from build123d import *

# Parameters (mm, degrees)
SKETCH1_R           = 5
BOSS_EXTRUDE1_DEPTH = 17
SKETCH2_R           = 5
SKETCH2_R_2         = 4
CUT_EXTRUDE1_DEPTH  = 12
CUT_EXTRUDE2_START  = -4
SKETCH3_R           = 4
SKETCH3_R_2         = 3.5
CUT_EXTRUDE2_DEPTH  = 1
SKETCH4_R           = 4
BOSS_EXTRUDE2_DEPTH = 6


with BuildPart() as part:
    # Sketch1 → Boss-Extrude1 (new, symmetric)
    with BuildSketch(Plane(origin=(0, 0, 0), x_dir=(1, 0, 0), z_dir=(0, 1, 0))):
        with Locations(Location((0, 0, 0), (0, 0, 270))):
            Circle(SKETCH1_R)
    extrude(amount=BOSS_EXTRUDE1_DEPTH, both=True)

    # Sketch2 → Cut-Extrude1 (cut)
    with BuildSketch(Plane(origin=(0, 17, 0), x_dir=(1, 0, 0), z_dir=(0, 1, 0))):
        with Locations(Location((0, 0, 0), (0, 0, 270))):
            Circle(SKETCH2_R)
        with Locations(Location((0, 0, 0), (0, 0, 270))):
            Circle(SKETCH2_R_2, mode=Mode.SUBTRACT)
    cut_extrude1 = extrude(amount=-CUT_EXTRUDE1_DEPTH, mode=Mode.SUBTRACT)

    # Mirror1: Cut-Extrude1 across plane
    add(cut_extrude1.mirror(Plane.ZX), mode=Mode.SUBTRACT)

    # Sketch3 → Cut-Extrude2 (cut)
    with BuildSketch(Plane(origin=(0, 17, 0), x_dir=(1, 0, 0), z_dir=(0, 1, 0)).offset(CUT_EXTRUDE2_START)):
        with Locations(Location((0, 0, 0), (0, 0, 270))):
            Circle(SKETCH3_R)
        with Locations(Location((0, 0, 0), (0, 0, 270))):
            Circle(SKETCH3_R_2, mode=Mode.SUBTRACT)
    cut_extrude2 = extrude(amount=-CUT_EXTRUDE2_DEPTH, mode=Mode.SUBTRACT)

    # Mirror2: Cut-Extrude2 across plane
    add(cut_extrude2.mirror(Plane.ZX), mode=Mode.SUBTRACT)

    # Sketch4 → Boss-Extrude2 (add)
    with BuildSketch(Plane(origin=(0, 17, 0), x_dir=(1, 0, 0), z_dir=(0, 1, 0))):
        with Locations(Location((0, 0, 0), (0, 0, 270))):
            Circle(SKETCH4_R)
    extrude(amount=BOSS_EXTRUDE2_DEPTH)


solid = part.part
Can you work these out from the model? Positions are in its coordinate system, mm. A direction names the side the tool comes from. Give positions to 0.01 mm unless a question says otherwise; leave off trailing zeros. Write each loop counter-clockwise with the first axis right and the second up, starting at its lowest first coordinate (ties: lowest second). Pieces come first, ordered by that corner, then holes. Notation, with made-up numbers: M 73,40.5 L 86,40.5 A19 ccw 86,71.5 Z; hole C 62.5,22 d6. An arc over 180 degrees is marked long. Answer in a Markdown table with one row per item. Add a question column.
Item 1: We'd pull the mould along Y, two halves only. Please class faces 1 (the cylindrical face through (-3.905, 8.549, -0.867)), 2 (the flat face through (0, -17, 0)), 3 (the cylindrical face through (-3.417, -12.507, -0.759)): released by +Y, released by -Y, zero draft, split by the parting line, or undercut.
Item 2: On a 3-axis mill with a long thin cutter (end or side, diameter ignored), from which of +Z, -Z, +X, -X, +Y, -Y can I reach the whole of each face in a straight line? I mean faces 4 (the cylindrical face through (-3.417, 12.507, -0.759)), 5 (the cylindrical face through (-3.905, -15.028, -0.867)), 6 (the cylindrical face through (-3.905, 17.93, -0.867)), 7 (the cylindrical face through (-4.88, 0.07, -1.08)), 8 (the flat face through (0, 23, 0)). Say none if no direction works.
Item 3: Imagine slicing it at D-D, the plane z = -4.5. Write out the boundary of the cut face in (x, y), plus the area to 3 significant figures.
Item 4: Imagine slicing it at C-C, the plane y = 7. Write out the boundary of the cut face in (x, z).
Item 5: Please list where these lines run through material, in increasing order: L1, parallel to Y at x = -2, z = 3.25; L2, parallel to Y at x = -1, z = 4.75; L3, parallel to Z at x = -3, y = 4.5.
Item 6: Imagine slicing it at B-B, the plane z = 0. Write out the boundary of the cut face in (x, y), plus the area to 3 significant figures.
Item 7: For pin 1 Ø1 at (x, y) = (-1, -8) entering from +Z; pin 2 Ø1 at (x, z) = (-3, -4) entering from +Y; pin 3 Ø2 at (x, y) = (0.5, -9) entering from -Z, each with a flat end and sliding along its axis, tell me the tip position at first contact or that it passes through.
Item 8: Imagine slicing it at A-A, the plane x = 0. Write out the boundary of the cut face in (y, z), plus the area to 3 significant figures.
Evaluation:
| question | item | result |
|---|---|---|
| 1 | face 1 | zero draft |
| 1 | face 2 | released by -Y |
| 1 | face 3 | undercut |
| 2 | face 4 | none |
| 2 | face 5 | -Y |
| 2 | face 6 | +Y |
| 2 | face 7 | +Y, -Y |
| 2 | face 8 | +Z, -Z, +X, -X, +Y |
| 3 | outline | M -2.18,-5 L 2.18,-5 L 2.18,5 L -2.18,5 Z |
| 3 | area | 43.6 mm² |
| 4 | outline | C 0,0 d8 |
| 5 | L1 | y = -17 to -13, -12 to 12, 13 to 23 |
| 5 | L2 | y = -5 to 5 |
| 5 | L3 | z = -4 to 4 |
| 6 | outline | M -5,-5 L -4,-5 L -4,-12 L -3.5,-12 L -3.5,-13 L -4,-13 L -4,-17 L 4,-17 L 4,-13 L 3.5,-13 L 3.5,-12 L 4,-12 L 4,-5 L 5,-5 L 5,5 L 4,5 L 4,12 L 3.5,12 L 3.5,13 L 4,13 L 4,23 L -4,23 L -4,13 L -3.5,13 L -3.5,12 L -4,12 L -4,5 L -5,5 Z |
| 6 | area | 338 mm² |
| 7 | pin 1 | stops at z = 3.97 |
| 7 | pin 2 | stops at y = 5 |
| 7 | pin 3 | stops at z = -4 |
| 8 | outline | M -17,-4 L -13,-4 L -13,-3.5 L -12,-3.5 L -12,-4 L -5,-4 L -5,-5 L 5,-5 L 5,-4 L 12,-4 L 12,-3.5 L 13,-3.5 L 13,-4 L 23,-4 L 23,4 L 13,4 L 13,3.5 L 12,3.5 L 12,4 L 5,4 L 5,5 L -5,5 L -5,4 L -12,4 L -12,3.5 L -13,3.5 L -13,4 L -17,4 Z |
| 8 | area | 338 mm² |
